Here's how the part is built. I have some questions about the finished solid (model axes, mm). A direction names the side the tool comes from. Coordinates: 2 decimals unless noted, no trailing zeros. Write each loop counter-clockwise with the first axis right and the second up, starting at its lowest first coordinate (ties: lowest second). Pieces come first, ordered by that corner, then holes. Notation, with made-up numbers: (81.5, 18.5) -> (99.5, 18.5) arc R15 cw to (99.5, 42.5) -> close; hole circle Ø7 at (-5, 57.25). An arc over 180 degrees is marked (long way). Put each result on its own line as item: value. Start each with the question number.
Item 1: I need wall thicknesses on line 1 (Y direction, x = 10, z = 7.5) (3 decimals); line 2 (Y direction, x = 12.3, z = 0) (3 decimals); line 3 (X direction, y = 4, z = -10). Which ranges of each line are inside material? Lowest first, please. Write a range as [from, to].
Item 2: For pin 1 (10 mm diameter, centred on x = 19, y = -8, fed in from +Z); pin 2 (1.5 mm diameter, centred on x = 11.5, y = 11, fed in from +Z); pin 3 (8 mm diameter, centred on x = 11, y = 9, fed in from +Z), each with a flat end and sliding along its axis, tell me the tip position at first contact or that it passes through.
Item 3: I want a section at C-C, the plane x = 3.25. List the corners of the cut face in (y, z) for me (3 decimals).
Item 4: I want a section at A-A, the plane x = 21. List the corners of the cut face in (y, z) for me (3 decimals).
Item 5: If we mould it in two halves opening along Y, with no side actions, what happens to faces 1 (the face through (0.386, -7.861, 13.359)), 2 (the face through (12.53, 7.83, 13.81)), 3 (the face through (13.462, 5.4, 2.4)), 4 (the face through (25.4, 10, -4))? For each: released by +Y, released by -Y, zero draft, split by the parting line, or undercut.
Item 6: On a 3-axis mill with a long thin cutter (end or side, diameter ignored), from which of +Z, -Z, +X, -X, +Y, -Y can I reach the whole of each face in a straight line? I mean faces 5 (the face through (25.146, -5, -5)), 6 (the face through (0.39, -7.64, -13.49)). Say none if no direction works.
from build123d import *

# Parameters (mm, degrees)
EXTRUDE1_DEPTH = 25.4
CHAMFER1_SIZE  = 0.254
CHAMFER2_SIZE  = 0.762
CHAMFER3_SIZE  = 0.762
CHAMFER4_SIZE  = 0.762


with BuildPart() as part:
    # Sketch1 → Extrude1 (new body)
    with BuildSketch(Plane(origin=(0, 0, 0), x_dir=(0, -1, 0), z_dir=(-1, 0, 0))):
        Polygon((15.875, 9.165435523), (0, 18.330871047), (-15.875, 9.165435523), (-15.875, -9.165435523), (0, -18.330871047), (15.875, -9.165435523), align=None)
    extrude(amount=-EXTRUDE1_DEPTH)

    # Sketch2 → Cut-Revolve1 (revolve, cut)
    with BuildSketch(Plane.XY, mode=Mode.PRIVATE) as cut_revolve1_sk:
        with BuildLine():
            Line((0, 11.8872), (0, 0))
            Line((0, 0), (25.4, 0))
            Line((25.4, 0), (25.4, 10.4775))
            Line((25.4, 10.4775), (25.146, 10.4775))
            Line((25.146, 10.4775), (25.146, 6.1849))
            Line((25.146, 6.1849), (22.5933, 5.642306865))
            Line((22.5933, 5.642306865), (21.929393135, 4.9784))
            Line((21.929393135, 4.9784), (13.462, 4.9784))
            Line((13.462, 4.9784), (13.462, 11.7221))
            Line((13.462, 11.7221), (10.16, 11.7221))
            ThreePointArc((10.16, 11.7221), (9.989969941, 11.844096333), (9.785188594, 11.8872))
            Line((9.785188594, 11.8872), (0, 11.8872))
        make_face()
    revolve(cut_revolve1_sk.sketch.rotate(Axis((0, 0, 0), (1, 0, 0)), 270), axis=Axis((0, 0, 0), (1, 0, 0)), mode=Mode.SUBTRACT)  # turned: the seam where the file's is

    # Chamfer1
    chamfer1_edges = [part.edges().sort_by_distance(p)[0] for p in [
        (0, 0, 11.8872),
    ]]
    chamfer(chamfer1_edges, length=CHAMFER1_SIZE)

    # Chamfer2
    chamfer2_edges = [part.edges().sort_by_distance(p)[0] for p in [
        (13.462, 0, 4.9784),
    ]]
    chamfer(chamfer2_edges, length=CHAMFER2_SIZE)

    # Chamfer3
    chamfer3_edges = [part.edges().sort_by_distance(p)[0] for p in [
        (0, -7.9375, -13.748153285),
        (0, 7.9375, -13.748153285),
        (0, 15.875, 0),
        (0, 7.9375, 13.748153285),
        (0, -7.9375, 13.748153285),
        (0, -15.875, 0),
    ]]
    chamfer(chamfer3_edges, length=CHAMFER3_SIZE)

    # Chamfer4
    chamfer4_edges = [part.edges().sort_by_distance(p)[0] for p in [
        (25.4, 7.9375, 13.748153285),
        (25.4, 15.875, 0),
        (25.4, 7.9375, -13.748153285),
        (25.4, -7.9375, -13.748153285),
        (25.4, -15.875, 0),
        (25.4, -7.9375, 13.748153285),
    ]]
    chamfer(chamfer4_edges, length=CHAMFER4_SIZE)


solid = part.part
Calculated:
1. line 1: y = [-15.875, -9.161], [9.161, 15.875]
1. line 2: y = [-15.875, -11.722], [11.722, 15.875]
1. line 3: x = [13.46, 25.4]
2. pin 1: stops at z = 16.6
2. pin 2: stops at z = 12.41
2. pin 3: stops at z = 15.44
3. outline: (-15.875, -9.165) -> (0, -18.331) -> (15.875, -9.165) -> (15.875, 9.165) -> (0, 18.331) -> (-15.875, 9.165) -> close; hole circle Ø23.774 at (0, 0)
4. outline: (-15.875, -9.165) -> (0, -18.331) -> (15.875, -9.165) -> (15.875, 9.165) -> (0, 18.331) -> (-15.875, 9.165) -> close; hole circle Ø9.957 at (0, 0)
5. face 1: released by -Y
5. face 2: released by +Y
5. face 3: undercut
5. face 4: zero draft
6. face 5: +X
6. face 6: -Z, -X, -Y
